Autodesk Inventor part; units mm, degrees
ref_plane "Arbeitsebene1" through (-6.0676, -4.4084, 330) normal (-0.809017, -0.5877853, 0) x (0.5877853, -0.809017, 0)
ref_plane "Arbeitsebene2" through (7.5, 0, 330) normal (1, 0, 0) x (0, 1, 0)
ref_plane "YZ Plane" through (0, 0, 0) normal (1, 0, 0) x (0, 1, 0)
sketch "Skizze1" plane through (0, 0, 0) normal (0, 0, 1) x (1, 0, 0)
  circle A0 centre (0, 0) radius 7.5
  dimension "d0" = 15
extrude "Extrusion1" add sketch "Skizze1" along normal blind 330
sketch "Skizze2" plane through (0, 0, 330) normal (0, 0, 1) x (1, 0, 0)
  point P0 (0, 0)
sketch "Skizze5" plane through (0, 0, 330) normal (0, 0, 1) x (1, 0, 0)
  line L0 (0, 0) -> (0, 2)
  line L1 (0, 2) -> (2, 2)
  line L2 (2, 2) -> (2, -2)
  line L3 (2, -2) -> (-2, -2)
  line L4 (-2, -2) -> (-2, 2)
  line L5 (-2, 2) -> (0, 2)
  dimension "d8" = 2
  dimension "d9" = 2
  dimension "d10" = 4
  dimension "d11" = 4
  dimension "d12" = 4
extrude "Extrusion4" add sketch "Skizze5" along normal blind 20
sketch "Skizze6" plane through (0, 0, 330) normal (0, 0, 1) x (1, 0, 0)
  line L0 (0, 0) -> (-6.0676, -4.4084)
  circle A0 centre (0, 0) radius 7.5
  line L1 (0, 0) -> (7.5, 0) construction
  line L2 (0, 0) -> (7.5, 0)
  line L3 (2, -2) -> (2, 2)
  dimension "d15" = 144
ref_plane "Arbeitsebene1" through (-6.0676, -4.4084, 330) normal (-0.809017, -0.5877853, 0) x (0.5877853, -0.809017, 0)
sketch "Skizze7" plane through (-6.0676, -4.4084, 330) normal (-0.809017, -0.5877853, 0) x (0.5877853, -0.809017, 0)
  line L0 (7.5, 0) -> (-7.5, 0)
  line L1 (0, 0) -> (0, -265)
  line L2 (-15, -336) -> (15, -336)
  point P0 (0, -330)
  dimension "d16" = 265
hole "Bohrung1" at (-6.0676, -4.4084, 65) direction (0.809017, 0.5877853, 0) diameter 3.2 depth 4 tip angle 118
ref_plane "Arbeitsebene2" through (7.5, 0, 330) normal (1, 0, 0) x (0, 1, 0)
sketch "Skizze8" plane through (7.5, 0, 330) normal (1, 0, 0) x (0, 1, 0)
  line L0 (7.5, 0) -> (-7.5, 0)
  line L1 (0, 0) -> (0, -265)
  point P0 (0, -330)
  dimension "d24" = 265
hole "Bohrung2" at (7.5, 0, 65) direction (-1, 0, 0) diameter 3.2 depth 4 tip angle 118
sketch "Skizze9" plane through (0, 0, 0) normal (0, 0, -1) x (-1, 0, 0)
  circle A0 centre (0, 0) radius 5
  circle A1 centre (0, 0) radius 7.5
  dimension "d32" = 10
extrude "Extrusion5" cut sketch "Skizze9" against normal blind 3
properties part number "Welle" material "Stahl"
The model under review builds one solid part; all positions refer to its coordinate system, in mm. A direction names the side the tool comes from. Round coordinates to 2 decimals unless told otherwise and drop trailing zeros. Loops run counter-clockwise (first coordinate to the right, second up) from the corner with the lowest first, then second, coordinate; pieces in that order, holes last. Notation, with made-up numbers: M -16.5,13 L 6.5,13 A30 ccw 6.5,38 Z; hole C -32.75,67 d2. An arc over 180 degrees is marked long. Answer as a JSON object with one key per item and string values.
(1) Take a section at A-A on z = 118.5. Give the boundary of the cut face in (x, y), and give its area (3 significant figures).
Resolved:
{"outline": "C 0,0 d15", "area": "177 mm²"}
(2) To check wall thickness, follow line 1 along Z through (x, y) = (4.5, 0); line 2 along Z through (x, y) = (5.2, 0); line 3 along Z through (x, y) = (-3.5, 1.25). State the ranges of each line that lie inside material, in increasing order.
Resolved:
{"line 1": "0 to 63.4, 66.6 to 330", "line 2": "3 to 63.4, 66.6 to 330", "line 3": "0 to 330"}
(3) Tool access review of faces 1 (the cylindrical face through (-7.493, -0.33, 164.211)), 2 (the cylindrical face through (1.08, -4.88, 1.48)): name each direction out of +Z, -Z, +X, -X, +Y, -Y from which nothing blocks a thin tool from reaching the whole face with its end or side.
Resolved:
{"face 1": "+Z, -Z", "face 2": "-Z"}
(4) Clearance check with flat-ended pins moving along their axes: P1, Ø3, axis at y = 0, z = 65, coming from the +X side; P2, Ø3, axis at y = 0.5, z = 339.5, coming from the -X side; P3, Ø3, axis at x = -3, y = -4.5, coming from the +Z side. State where each tip first meets the part, or that it passes through.
Resolved:
{"P1": "x = 3.44", "P2": "x = -2", "P3": "z = 330"}
